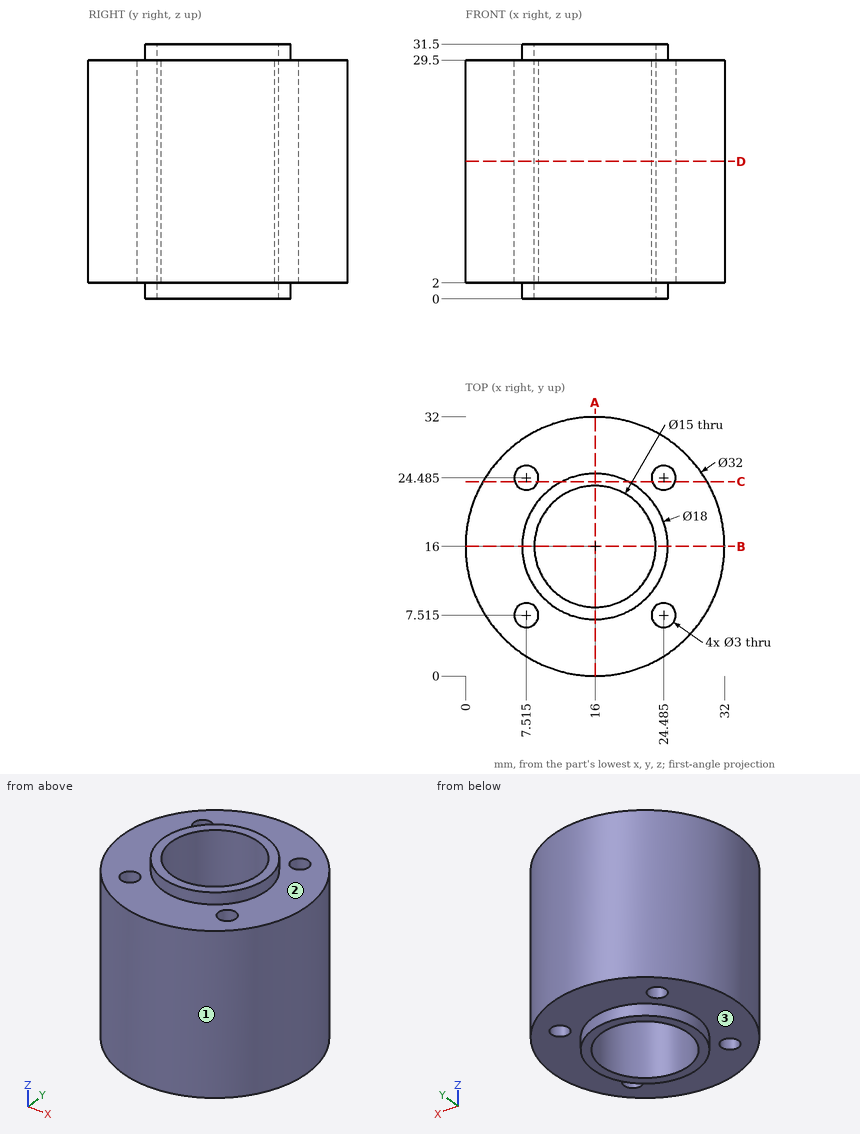
The figure shows three views and two pictorial views of one solid part (mm, origin at its lowest corner). Answer the questions. A direction names the side the tool comes from. Coordinates: 2 decimals unless noted, no trailing zeros. Loops run counter-clockwise (first coordinate to the right, second up) from the corner with the lowest first, then second, coordinate; pieces in that order, holes last. Notation, with made-up numbers: (-6.5, 77.5) -> (49.5, 77.5) arc R27 ccw to (49.5, 110.5) -> close; hole circle Ø5 at (65, 32). An arc over 180 degrees is marked (long way). Use one line per item in the form item = value. Start each with the question number.
Item 1: A tool of negligible diameter and unlimited length cuts with its end or side. For the marked faces 1, 2 and 3, from which of +Z, -Z, +X, -X, +Y, -Y can it reach the whole face along a straight path? Write none if from no direction.
Item 2: The part is cut by section A-A on x = 16. Determine the outline of the cut face in (y, z).
Item 3: The part is cut by section C-C on y = 24. Determine the outline of the cut face in (x, z) (1 decimal).
Item 4: Consider L1, parallel to Y at x = 8, z = 7 (1 decimal); L2, parallel to Z at x = 27.5, y = 14. Determine where each line is inside the solid, lowest interval first. Write a range as [from, to].
Item 5: The part is cut by section D-D on z = 17. Determine the outline of the cut face in (x, y) (1 decimal).
Item 6: Flat-ended cylindrical pins translate along their axes: pin 1 Ø2.5 at (x, y) = (24.49, 24.49) entering from -Z; pin 2 Ø8 at (x, z) = (13, 4.5) entering from -Y; pin 3 Ø4 at (x, z) = (19.5, 25) entering from +Y; pin 4 Ø12 at (x, z) = (4, 12.5) entering from -Y. Find the tip coordinate at first contact, or state that the pin passes through.
Answer key:
q1.face_1 = +Z, -Z
q1.face_2 = +Z
q1.face_3 = -Z
q2.outline = (0, 2) -> (7, 2) -> (7, 0) -> (8.5, 0) -> (8.5, 31.5) -> (7, 31.5) -> (7, 29.5) -> (0, 29.5) -> close; (23.5, 0) -> (25, 0) -> (25, 2) -> (32, 2) -> (32, 29.5) -> (25, 29.5) -> (25, 31.5) -> (23.5, 31.5) -> close
q3.outline = (2.1, 2) -> (6.1, 2) -> (6.1, 29.5) -> (2.1, 29.5) -> close; (8.9, 2) -> (11.9, 2) -> (11.9, 0) -> (20.1, 0) -> (20.1, 2) -> (23.1, 2) -> (23.1, 29.5) -> (20.1, 29.5) -> (20.1, 31.5) -> (11.9, 31.5) -> (11.9, 29.5) -> (8.9, 29.5) -> close; (25.9, 2) -> (29.9, 2) -> (29.9, 29.5) -> (25.9, 29.5) -> close
q4.L1 = [2.1, 6.1], [8.9, 23.1], [25.9, 29.9]
q4.L2 = [2, 29.5]
q5.outline = circle Ø32 at (16, 16); hole circle Ø3 at (7.5, 7.5); hole circle Ø3 at (7.5, 24.5); hole circle Ø15 at (16, 16); hole circle Ø3 at (24.5, 7.5); hole circle Ø3 at (24.5, 24.5)
q6.pin_1 = through
q6.pin_2 = 0
q6.pin_3 = 31.93
q6.pin_4 = 1.17
